Source: CAD feature listing. Evaluate the final solid. Frame: model axes, mm. Face numbers are marked on the shaded views. A direction names the side the tool comes from. Round coordinates to 2 decimals unless told otherwise and drop trailing zeros. Write each loop counter-clockwise with the first axis right and the second up, starting at its lowest first coordinate (ties: lowest second). Pieces come first, ordered by that corner, then holes. Notation, with made-up numbers: M -2.75,23.25 L 18.25,23.25 A21 cw 18.25,31.25 Z; hole C 35,12 d5. An arc over 180 degrees is marked long. Answer in a Markdown table with one row per item. Add a question column.
Item 1: Cut plane B-B on x = 9. Return loops of the section in (y, z), and give its area (3 significant figures).
Item 2: Cut plane A-A on y = 0. Return loops of the section in (x, z), and give its area (3 significant figures).
Item 3: Contact query for flat-ended pins moving along their axis: pin 1 (2 mm diameter, centred on y = 16.5, z = 44, fed in from +X); pin 2 (3 mm diameter, centred on y = 12, z = 56, fed in from -X); pin 3 (6 mm diameter, centred on x = 15.5, z = 62, fed in from -Y). Output: stop coordinate, or through.
Item 4: Set-up query: the marked faces 1, 2, 3, 4 and 5. Return all of +Z, -Z, +X, -X, +Y, -Y with unobstructed straight access to the full face (end or side cutting, diameter ignored); none if empty.
Item 5: Mould query, pull axis Y, two halves, no side actions, for the marked faces 6, 7, 8 and 9. Classes: released by +Y, released by -Y, zero draft, split by the parting line, or undercut.
Item 6: Cut plane D-D on y = 12.5. Return loops of the section in (x, z), and give its area (3 significant figures).
Item 7: Cut plane C-C on z = -5. Return loops of the section in (x, y), and give its area (3 significant figures).
Item 8: Material intervals for probe 1 along Z at (x, y) = (13, 0); probe 2 along Y at (x, z) = (-8.5, 54); probe 3 along Z at (x, y) = (7.5, 11.5), sorted ascending.
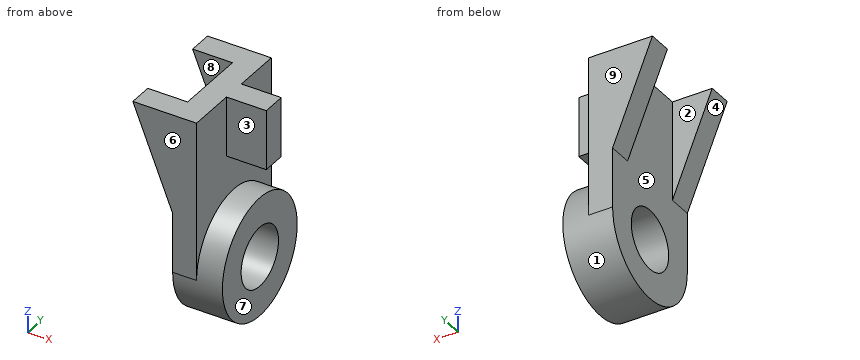
from build123d import *

# Parameters (mm, degrees)
BOSS_EXTRUDE1_DEPTH     = 12
SKETCH1_3_R             = 30
BOSS_EXTRUDE2_DEPTH     = 25
SKETCH2_W               = 20
SKETCH2_H               = 30
BOSS_EXTRUDE3_DEPTH     = 6
BOSS_EXTRUDE4_DEPTH     = 12
CUT_EXTRUDE1_DEPTH      = 97.566039579
CUT_EXTRUDE1_DEPTH_BACK = 97.566039579
SKETCH4_R               = 15


with BuildPart() as part:
    # Sketch1 → Boss-Extrude1 (new body)
    with BuildSketch(Plane.YZ):
        with BuildLine():
            Line((-30, 80), (-30, 0))
            ThreePointArc((-30, 0), (0, 30), (30, 0))
            Line((30, 0), (30, 80))
            Line((30, 80), (-30, 80))
        make_face()
    extrude(amount=BOSS_EXTRUDE1_DEPTH)

    # Sketch1_3 → Boss-Extrude2 (add)
    with BuildSketch(Plane.YZ):
        Circle(SKETCH1_3_R)
    extrude(amount=BOSS_EXTRUDE2_DEPTH)

    # Sketch2 → Boss-Extrude3 (add, symmetric)
    with BuildSketch(Plane(origin=(0, 0, 0), x_dir=(-1, 0, 0), z_dir=(0, 1, 0))):
        with Locations((-22, 65)):
            Rectangle(SKETCH2_W, SKETCH2_H)
    extrude(amount=BOSS_EXTRUDE3_DEPTH, both=True)

    # Sketch3 → Boss-Extrude4 (add)
    with BuildSketch(Plane(origin=(0, 30, 0), x_dir=(-1, 0, 0), z_dir=(0, 1, 0))):
        Polygon((0, 80), (20, 80), (0, 30), align=None)
    boss_extrude4 = extrude(amount=-BOSS_EXTRUDE4_DEPTH)

    # Mirror1: Boss-Extrude4 across plane
    add(boss_extrude4.mirror(Plane.ZX))

    # Sketch4 → Cut-Extrude1 (cut, two sides: drawn at the far end of the back side and taken through both)
    with BuildSketch(Plane.YZ.offset(25).offset(-CUT_EXTRUDE1_DEPTH_BACK)):
        with Locations(Location((0, 0, 0), (0, 0, 270))):
            Circle(SKETCH4_R)
    extrude(amount=CUT_EXTRUDE1_DEPTH + CUT_EXTRUDE1_DEPTH_BACK, mode=Mode.SUBTRACT)


solid = part.part
Results below:
| question | item | result |
|---|---|---|
| 1 | outline | M -30,0 A30 ccw 30,0 L 30,80 L -30,80 Z; hole C 0,0 d30 |
| 1 | area | 5,510 mm2 |
| 2 | outline | M 0,-30 L 25,-30 L 25,-15 L 0,-15 Z; M 0,15 L 25,15 L 25,30 L 12,30 L 12,50 L 32,50 L 32,80 L 0,80 Z |
| 2 | area | 1,950 mm2 |
| 3 | pin 1 | x = 12 |
| 3 | pin 2 | x = 0 |
| 3 | pin 3 | y = -6 |
| 4 | face 1 | +X |
| 4 | face 2 | +Z, -Z, -X |
| 4 | face 3 | +Z, +X, -Y |
| 4 | face 4 | -Z, -X, +Y, -Y |
| 4 | face 5 | -Z, -X |
| 5 | face 6 | released by -Y |
| 5 | face 7 | zero draft |
| 5 | face 8 | undercut |
| 5 | face 9 | released by +Y |
| 6 | outline | M 0,-27.27 L 25,-27.27 L 25,-8.29 L 0,-8.29 Z; M 0,8.29 L 25,8.29 L 25,27.27 L 12,27.27 L 12,80 L 0,80 Z |
| 6 | area | 1,580 mm2 |
| 7 | outline | M 0,-29.58 L 25,-29.58 L 25,-14.14 L 0,-14.14 Z; M 0,14.14 L 25,14.14 L 25,29.58 L 0,29.58 Z |
| 7 | area | 772 mm2 |
| 8 | probe 1 | -30 to -15, 15 to 30, 50 to 80 |
| 8 | probe 2 | -30 to -18, 18 to 30 |
| 8 | probe 3 | -27.71 to -9.63, 9.63 to 80 |
